Read the model definition and answer for the solid it produces. Units are mm, in the model's axes. Give positions to 0.01 mm unless a question says otherwise; leave off trailing zeros. Loops run counter-clockwise (first coordinate to the right, second up) from the corner with the lowest first, then second, coordinate; pieces in that order, holes last. Notation, with made-up numbers: (40, 89) -> (58, 89) arc R23 ccw to (58, 128) -> close; hole circle Ø9 at (57.5, 76.25). An arc over 180 degrees is marked (long way). Return JSON: item names as keys, results as strings. Group by question number.
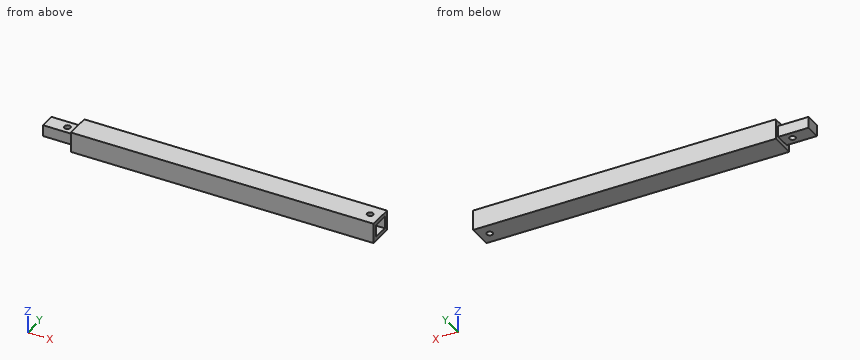
Autodesk Fusion 360 part; units mm, degrees
sketch "Sketch1" plane through (0, 0, 0) normal (0, 0, 1) x (1, 0, 0)
  line L0 (0, 0) -> (150, 0)
  line L1 (150, 0) -> (150, -12)
  line L2 (150, -12) -> (0, -12)
  line L3 (0, -12) -> (0, 0)
  dimension "d16" = 150
  dimension "d17" = 12
extrude "Extrude1" add sketch "Sketch1" along normal blind 10
sketch "Sketch3" plane through (0, 0, 0) normal (-1, 0, 0) x (0, -1, 0)
  line L0 (0, 0) -> (12, 0)
  line L1 (12, 0) -> (12, 10)
  line L2 (12, 10) -> (0, 10)
  line L3 (0, 10) -> (0, 0)
  line L4 (2.2, 7.8) -> (9.8, 7.8)
  line L5 (9.8, 7.8) -> (9.8, 2.2)
  line L6 (9.8, 2.2) -> (2.2, 2.2)
  line L7 (2.2, 2.2) -> (2.2, 7.8)
  dimension "d22" = 7.6
  dimension "d23" = 5.6
  dimension "d26" = 2.2
  dimension "d27" = 2.2
extrude "Extrude2" add sketch "Sketch3" along normal blind 15 contours L4 L5 L6 L7
sketch "Sketch4" plane through (150, 0, 0) normal (1, 0, 0) x (0, 1, 0)
  line L0 (-12, 0) -> (0, 0)
  line L1 (0, 0) -> (0, 10)
  line L2 (0, 10) -> (-12, 10)
  line L3 (-12, 10) -> (-12, 0)
  line L4 (-10, 8) -> (-2, 8)
  line L5 (-2, 8) -> (-2, 2)
  line L6 (-2, 2) -> (-10, 2)
  line L7 (-10, 2) -> (-10, 8)
  dimension "d30" = 6
  dimension "d31" = 8
  dimension "d34" = 2
  dimension "d35" = 2
extrude "Extrude3" cut sketch "Sketch4" against normal blind 15 contours L4 L5 L6 L7
sketch "Sketch5" plane through (0, 0, 7.8) normal (0, 0, 1) x (-1, 0, 0)
  line L0 (0, 2.2) -> (15, 2.2)
  line L1 (15, 2.2) -> (15, 9.8)
  line L2 (15, 9.8) -> (0, 9.8)
  circle A0 centre (5, 6) radius 1.5
  circle A1 centre (-145, 6) radius 1.5
  line L3 (-150, 12) -> (-150, 0)
  line L4 (-150, 0) -> (0, 0)
  line L5 (0, 9.8) -> (0, 2.2)
  dimension "d37" = 3
  dimension "d38" = 3
  dimension "d43" = 10
  dimension "d44" = 3.8
  dimension "d45" = 5
  dimension "d46" = 6
extrude "Extrude4" cut sketch "Sketch5" against normal blind 100 contours A0
extrude "Extrude5" cut sketch "Sketch5" along normal mid plane 200 contours A1
equation "main_length = 150 mm"
equation "height = 10 mm"
equation "dowel_edge_width = 7.6 mm"
equation "dowel_edge_length = 15 mm"
equation "length = 180 mm"
equation "edge_hole_radius = 1.5 mm"
equation "dowel_edge_hole_big_distance = 10 mm"
equation "dowel_edge_hole_small_distance = dowel_edge_width / 2"
equation "hollow_edge_length = 15 mm"
equation "hollow_edge_width = 8 mm"
equation "width = 12 mm"
equation "dowel_edge_height = 5.6 mm"
equation "hollow_edge_height = 6 mm"
equation "hollow_edge_hole_big_distance = 5 mm"
equation "hollow_edge_hole_small_distance = width / 2"
equation "d16 = main_length"
equation "d17 = width"
equation "d18 = height"
equation "dowel_edge_small_distance = ( width - dowel_edge_width ) / 2"
equation "dowel_edge_big_distance = ( height - dowel_edge_height ) / 2"
equation "d22 = dowel_edge_width"
equation "d23 = dowel_edge_height"
equation "d24 = dowel_edge_length"
equation "d26 = dowel_edge_big_distance"
equation "d27 = dowel_edge_small_distance"
equation "hollow_edge_small_distance = ( width - hollow_edge_width ) / 2"
equation "hollow_edge_big_distance = ( height - hollow_edge_height ) / 2"
equation "d30 = hollow_edge_height"
equation "d31 = hollow_edge_width"
equation "d34 = hollow_edge_big_distance"
equation "d35 = hollow_edge_small_distance"
equation "extra = 100 mm"
equation "d37 = edge_hole_radius * 2"
equation "d38 = edge_hole_radius * 2"
equation "d41 = extra"
equation "d43 = dowel_edge_hole_big_distance"
equation "d44 = dowel_edge_hole_small_distance"
equation "d45 = hollow_edge_hole_big_distance"
equation "d46 = hollow_edge_hole_small_distance"
1. Section B-B on y = -6 is taken. Determine the outline of the cut face in (x, z).
2. Section D-D on x = -5 is taken. Determine the outline of the cut face in (y, z).
3. Section C-C on z = 4.25 is taken. Determine the outline of the cut face in (x, y), then the cut area to 3 significant figures.
4. Flat-ended cylindrical pins translate along their axes: pin 1 Ø4 at (x, y) = (-5, -6) entering from +Z; pin 2 Ø1.7 at (x, z) = (-10.5, 5) entering from -Y; pin 3 Ø6 at (x, y) = (-11, -4.5) entering from -Z. Find the tip coordinate at first contact, or state that the pin passes through.
5. Section A-A on x = 145 is taken. Determine the outline of the cut face in (y, z), then the cut area to 3 significant figures.
6. Straight lines are drawn through the part: line 1 (X direction, y = -6, z = 6.2); line 2 (Y direction, x = -5, z = 4.8); line 3 (Y direction, x = 145, z = 0.8). For each, find the intervals that lie inside material, in ascending order. Write a range as from..to.
Completed:
{
 "1": {"outline": "(-15, 2.2) -> (-6.5, 2.2) -> (-6.5, 7.8) -> (-15, 7.8) -> close; (-3.5, 2.2) -> (0, 2.2) -> (0, 0) -> (143.5, 0) -> (143.5, 2) -> (135, 2) -> (135, 8) -> (143.5, 8) -> (143.5, 10) -> (0, 10) -> (0, 7.8) -> (-3.5, 7.8) -> close; (146.5, 0) -> (150, 0) -> (150, 2) -> (146.5, 2) -> close; (146.5, 8) -> (150, 8) -> (150, 10) -> (146.5, 10) -> close"},
 "2": {"outline": "(-9.8, 2.2) -> (-7.5, 2.2) -> (-7.5, 7.8) -> (-9.8, 7.8) -> close; (-4.5, 2.2) -> (-2.2, 2.2) -> (-2.2, 7.8) -> (-4.5, 7.8) -> close"},
 "3": {"outline": "(-15, -9.8) -> (0, -9.8) -> (0, -12) -> (150, -12) -> (150, -10) -> (135, -10) -> (135, -2) -> (150, -2) -> (150, 0) -> (0, 0) -> (0, -2.2) -> (-15, -2.2) -> close; hole circle Ø3 at (-5, -6)", "area": "1,790 mm²"},
 "4": {"pin 1": "stops at z = 7.8", "pin 2": "stops at y = -9.8", "pin 3": "stops at z = 2.2"},
 "5": {"outline": "(-12, 0) -> (-7.5, 0) -> (-7.5, 2) -> (-10, 2) -> (-10, 8) -> (-7.5, 8) -> (-7.5, 10) -> (-12, 10) -> close; (-4.5, 0) -> (0, 0) -> (0, 10) -> (-4.5, 10) -> (-4.5, 8) -> (-2, 8) -> (-2, 2) -> (-4.5, 2) -> close", "area": "60.0 mm²"},
 "6": {"line 1": "x = -15..-6.5, -3.5..135", "line 2": "y = -9.8..-7.5, -4.5..-2.2", "line 3": "y = -12..-7.5, -4.5..0"}
}
